Answer from the drawing. Dimensions are ordinates in mm from the lowest x, y and z of the part. Give positions to 0.01 mm unless a question says otherwise; leave off trailing zeros. Order: outer loops, then holes, each group sorted by start corner. A loop starts at its lowest first (then second) coordinate and runs counter-clockwise, first axis right, second up. Notation, with made-up numbers: (66, 17) -> (83, 17) arc R15 ccw to (83, 36) -> close; hole circle Ø8 at (1.5, 11.5). An arc over 180 degrees is marked (long way). Answer as a JSON object with one key per item and string values. Group by question number.
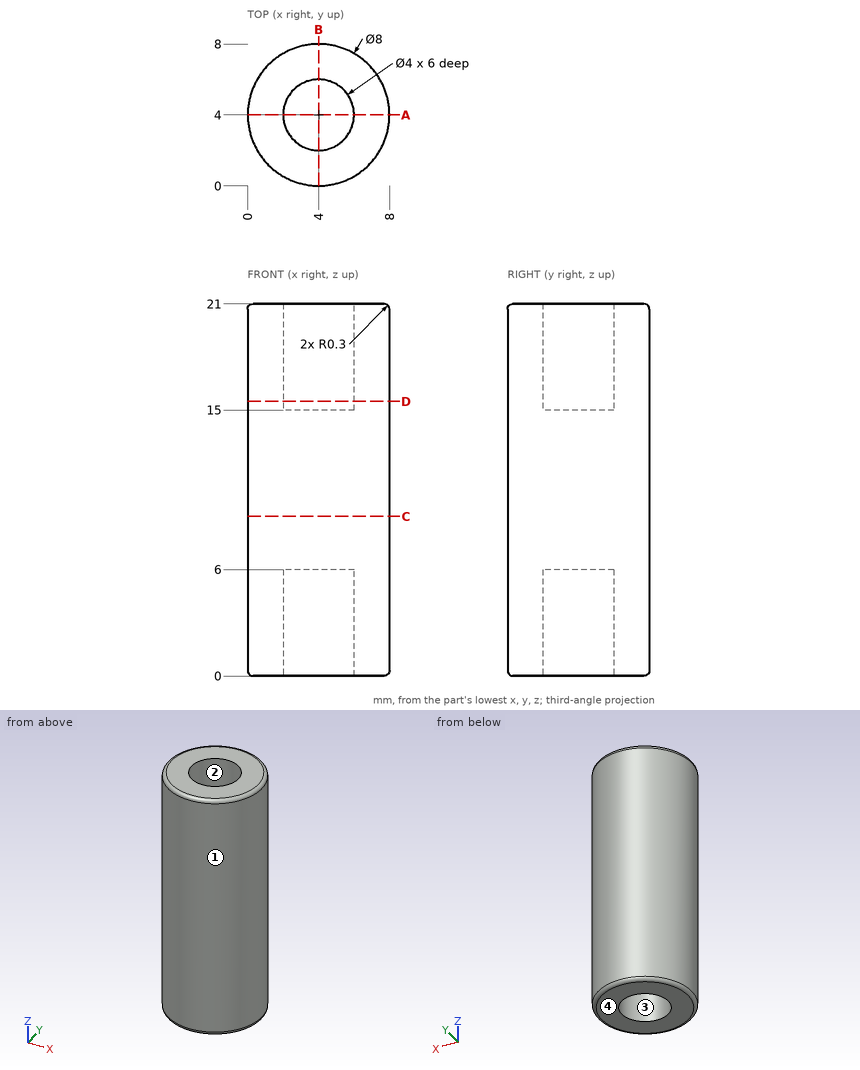
(1) A cutting plane is placed at A-A (y = 4). Determine the outline of the cut face in (x, z).
(2) A cutting plane is placed at C-C (z = 9). Determine the outline of the cut face in (x, y).
(3) A cutting plane is placed at D-D (z = 15.5). Determine the outline of the cut face in (x, y).
(4) For a pull along X with two mould halves and no side action, classify the marked faces 1, 2, 3 and 4 as +X half, -X half, draft (parallel to the pull), parting line (faces both ways), or undercut.
(5) Find the intervals of material crossed by line 1 along Y through (x, z) = (4, 1.35); line 2 along Z through (x, y) = (3, 5); line 3 along Y through (x, z) = (3, 18.25), in increasing order. Write a range as [from, to].
(6) Flat-ended cylindrical pins translate along their axes: pin 1 Ø1.2 at (x, y) = (4, 3) entering from -Z; pin 2 Ø2 at (y, z) = (2.5, 11.5) entering from +X; pin 3 Ø2.5 at (x, y) = (4, 4) entering from +Z. Find the tip coordinate at first contact, or state that the pin passes through.
Check sheet entries:
{
 "1": {"outline": "(0, 0.3) arc R0.3 ccw to (0.3, 0) -> (2, 0) -> (2, 6) -> (6, 6) -> (6, 0) -> (7.7, 0) arc R0.3 ccw to (8, 0.3) -> (8, 20.7) arc R0.3 ccw to (7.7, 21) -> (6, 21) -> (6, 15) -> (2, 15) -> (2, 21) -> (0.3, 21) arc R0.3 ccw to (0, 20.7) -> close"},
 "2": {"outline": "circle Ø8 at (4, 4)"},
 "3": {"outline": "circle Ø8 at (4, 4); hole circle Ø4 at (4, 4)"},
 "4": {"face 1": "parting line", "face 2": "undercut", "face 3": "undercut", "face 4": "draft"},
 "5": {"line 1": "y = [0, 2], [6, 8]", "line 2": "z = [6, 15]", "line 3": "y = [0.13, 2.27], [5.73, 7.87]"},
 "6": {"pin 1": "stops at z = 6", "pin 2": "stops at x = 7.97", "pin 3": "stops at z = 15"}
}
